from build123d import *

# Parameters (mm, degrees)
F2_DEPTH = 12.7
F3_DEPTH = 25.4


# Not quite as in the source:
# - a feature names something its author has since deleted; it is built from what else it names


with BuildPart() as f2:
    # F0 (on Front) → F2 (new body, symmetric)
    with BuildSketch(Plane.XZ):
        Polygon((22.225, 9.525), (-41.275, 9.525), (-41.275, -9.525), (41.275, -9.525), (41.275, 9.525), align=None)
    extrude(amount=F2_DEPTH, both=True)

    # F0 (on Front) → F3 (join)
    with BuildSketch(Plane.XZ):
        with BuildLine():
            add(Edge.make_bspline(
                [(-41.275, 9.525), (-40.7984927297, 44.0375059843), (14.3764037639, 61.959747225), (57.15, 61.9252)],
                knots=[0, 0, 0, 0, 111.5045361635, 111.5045361635, 111.5045361635, 111.5045361635], degree=3))
            Line((-41.275, 9.525), (22.225, 9.525))
            Line((22.225, 9.525), (22.225, 27.0002))
            ThreePointArc((22.225, 27.0002), (32.4542956671, 51.6959043329), (57.15, 61.9252))
        make_face()
        Polygon((22.225, 9.525), (-41.275, 9.525), (-41.275, -9.525), (41.275, -9.525), (41.275, 9.525), align=None)
        with BuildLine():
            Line((22.225, 27.0002), (22.225, 9.525))
            Line((22.225, 9.525), (41.275, 9.525))
            Line((41.275, 9.525), (41.275, 27.0002))
            ThreePointArc((41.275, 27.0002), (45.9246798487, 38.2255201513), (57.15, 42.8752))
            Line((57.15, 42.8752), (60.325, 42.8752))
            Line((60.325, 42.8752), (60.325, 61.9252))
            Line((60.325, 61.9252), (57.15, 61.9252))
            ThreePointArc((57.15, 61.9252), (32.4542956671, 51.6959043329), (22.225, 27.0002))
        make_face()
        Polygon((74.2425137572, 61.9252), (60.325, 61.9252), (60.325, 42.8752), (74.2425137572, 42.8752), (85.725, 42.8752), (85.725, 61.9252), align=None)
        Polygon((60.325, 66.675), (60.325, 61.9252), (74.2425137572, 61.9252), (85.725, 61.9252), (85.725, 66.675), align=None)
        Polygon((74.2425137572, 42.8752), (60.325, 42.8752), (60.325, 38.1), (85.725, 38.1), (85.725, 42.8752), align=None)
        Polygon((111.125, 66.675), (85.725, 66.675), (85.725, 61.9252), (85.725, 42.8752), (85.725, 38.1), (111.125, 38.1), align=None)
    extrude(amount=F3_DEPTH)


solid = f2.part
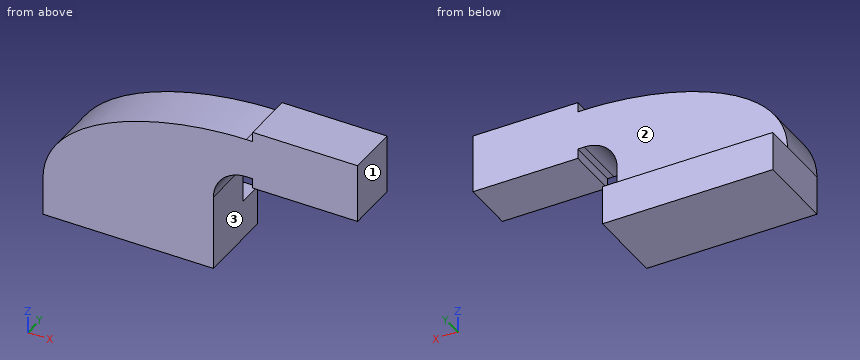
Design review of the part built by this model. Coordinates are the model's own, in mm. Face numbers are marked on the shaded views. A direction names the side the tool comes from. Give positions to 0.01 mm unless a question says otherwise; leave off trailing zeros. Loops run counter-clockwise (first coordinate to the right, second up) from the corner with the lowest first, then second, coordinate; pieces in that order, holes last. Notation, with made-up numbers: M 6,-23.75 L 53,-23.75 A26 ccw 53,0.25 Z; hole C 58,-8.75 d11. An arc over 180 degrees is marked long. Answer as a JSON object with one key per item and string values.
Item 1: Wall thickness on line 1 along X through (y, z) = (-14.5, 6) (3 decimals); line 2 along Z through (x, y) = (-22.5, 11) (3 decimals); line 3 along Y through (x, z) = (22, 38.5): over which ranges is each line inside the solid? List them lowest first.
Output values:
{"line 1": "x = -41.275 to 41.275", "line 2": "z = -9.525 to 9.525", "line 3": "y = -25.4 to 0"}
Item 2: Machinability: for the marked faces 1, 2 and 3, which of the approach directions +Z, -Z, +X, -X, +Y, -Y give a long, thin tool a straight path to every point of the face, cutting with its end or side? Answer none if there is none.
Output values:
{"face 1": "+Z, -Z, +X, +Y, -Y", "face 2": "+Z, +X, -X, +Y", "face 3": "-Z, +X, +Y, -Y"}
Item 3: For P1, Ø11, axis at y = -13.5, z = 7, coming from the +X side (3 decimals); P2, Ø3, axis at y = -19.5, z = 36.5, coming from the -X side; P3, Ø4, axis at x = 17, y = 7, coming from the +Z side (3 decimals); P4, Ø2, axis at y = 2.5, z = 59, coming from the -X side, all flat-tipped, find the tip position at first contact; note any pin that passes through.
Output values:
{"P1": "stops at x = 41.275", "P2": "stops at x = -29.05", "P3": "stops at z = 9.525", "P4": "passes through"}
Item 4: We need section B-B (z = 7). State the section outline as (x, y) points (3 decimals).
Output values:
{"outline": "M -41.275,-25.4 L 41.275,-25.4 L 41.275,12.7 L -41.275,12.7 Z"}
Item 5: We need section A-A (y = 7). State the section outline as (x, z) points (3 decimals), and give its area (3 significant figures).
Output values:
{"outline": "M -41.275,-9.525 L 41.275,-9.525 L 41.275,9.525 L -41.275,9.525 Z", "area": "1,570 mm2"}
